The model under review builds one solid part; all positions refer to its coordinate system, in mm. A direction names the side the tool comes from. Give positions to 0.01 mm unless a question says otherwise; leave off trailing zeros. Loops run counter-clockwise (first coordinate to the right, second up) from the corner with the lowest first, then second, coordinate; pieces in that order, holes last. Notation, with made-up numbers: M 81.5,38.25 L 123.5,38.25 A11 ccw 123.5,57.25 Z; hole C 56,26.5 d1. An arc over 180 degrees is marked long. Return JSON: item names as keys, results as strings.
```python
from build123d import *

# Parameters (mm, degrees)
F0_W     = 15
F0_H     = 15
F1_DEPTH = 15
F3_DEPTH = 10


with BuildPart() as f1:
    # F0 (on Top) → F1 (new body)
    with BuildSketch(Plane.XY):
        with Locations((5.322702, 2.974191)):
            Rectangle(F0_W, F0_H)
    extrude(amount=F1_DEPTH)

    # F2 (on face) → F3 (join)
    with BuildSketch(Plane.XZ.offset(4.525809)):
        Polygon((12.822702, 0), (12.822702, 10), (2.822702, 0), align=None)
    extrude(amount=F3_DEPTH)


solid = f1.part
```
1) Consider section A-A on z = 1.5. Write out the cut boundary in (x, y).
From the geometry:
{"outline": "M -2.18,-4.53 L 4.32,-4.53 L 4.32,-14.53 L 12.82,-14.53 L 12.82,10.47 L -2.18,10.47 Z"}
2) Insertion check: pin 1 (4 mm diameter, centred on x = 10.5, y = -11.5, fed in from +Z); pin 2 (4 mm diameter, centred on x = 1.5, y = -5.5, fed in from +Z); pin 3 (1 mm diameter, centred on x = 4, z = 4, fed in from -Y). Each pin has a flat end and moves straight along its axis. Give the tip position at first contact, or say it passes through.
From the geometry:
{"pin 1": "z = 9.68", "pin 2": "z = 15", "pin 3": "y = -4.53"}
3) Consider section B-B on x = 7.5. Write out the cut boundary in (y, z), then the cut area to 3 significant figures.
From the geometry:
{"outline": "M -14.53,0 L 10.47,0 L 10.47,15 L -4.53,15 L -4.53,4.68 L -14.53,4.68 Z", "area": "272 mm²"}
4) Consider section D-D on z = 11.5. Write out the cut boundary in (x, y), then the cut area to 3 significant figures.
From the geometry:
{"outline": "M -2.18,-4.53 L 12.82,-4.53 L 12.82,10.47 L -2.18,10.47 Z", "area": "225 mm²"}
5) Tool access review of faces 1 (the face through (10, -14.526, 3)), 2 (the face through (7.89, -9.46, 5.07)): name each direction out of +Z, -Z, +X, -X, +Y, -Y from which nothing blocks a thin tool from reaching the whole face with its end or side.
From the geometry:
{"face 1": "+Z, -Z, +X, -X, -Y", "face 2": "+Z, -X, -Y"}
6) Consider section C-C on y = -5. Write out the cut boundary in (x, z), then the cut area to 3 significant figures.
From the geometry:
{"outline": "M 2.82,0 L 12.82,0 L 12.82,10 Z", "area": "50.0 mm²"}
7) Wall thickness on L1, parallel to Y at x = 5.25, z = 4.5; L2, parallel to X at y = -11, z = 8.75; L3, parallel to Z at x = 12.25, y = -8: over which ranges is each line inside the solid? List them lowest first. Write a range as from..to.
From the geometry:
{"L1": "-4.53..10.47", "L2": "11.57..12.82", "L3": "0..9.43"}
